Can you work these out from the model? Positions are in its coordinate system, mm. Face numbers are marked on the shaded views. A direction names the side the tool comes from. Give positions to 0.01 mm unless a question says otherwise; leave off trailing zeros. Loops run counter-clockwise (first coordinate to the right, second up) from the corner with the lowest first, then second, coordinate; pieces in that order, holes last. Notation, with made-up numbers: (-33.75, 60.25) - (-17.75, 60.25) arc R16 ccw to (-17.75, 84.25) - close; hole circle Ø3 at (-25.5, 88.25). An arc over 180 degrees is marked (long way). Answer as a JSON object with one key per item and string values. Group by question number.
Item 1: Will these pins go through, and if not, where does the flat tip stop? pin 1 (3 mm diameter, centred on y = 7.5, z = -3.5, fed in from -X); pin 2 (5 mm diameter, centred on x = 14.351, z = 0, fed in from -Y); pin 3 (1 mm diameter, centred on x = -2.5, y = 4, fed in from -Z); pin 4 (2 mm diameter, centred on y = 5.5, z = 5, fed in from +X).
Item 2: Suppose I cut it at C-C on y = 1.5. Count the separate pieces of the cut face and the enclosed holes in it, and give its area (3 significant figures).
Item 3: Please list where these lines run through material, in increasing order: L1, parallel to X at y = 3.75, z = 0; L2, parallel to X at y = 10, z = 6.5; L3, parallel to X at y = 1.5, z = 1.
Item 4: Which directions (+Z, -Z, +X, -X, +Y, -Y) give clear straight access to the entire face, cutting with the end or side of a thin tool? Please do the marked faces 1, 2 and 3.
Item 5: Suppose I cut it at D-D on z = 4. Write out the boundary of the cut face in (x, y), and give its area (3 significant figures).
Item 6: Suppose I cut it at A-A on z = 0. Write out the boundary of the cut face in (x, y), and give its area (3 significant figures).
Item 7: Suppose I cut it at B-B on x = -14. Write out the boundary of the cut face in (y, z), and give its area (3 significant figures).
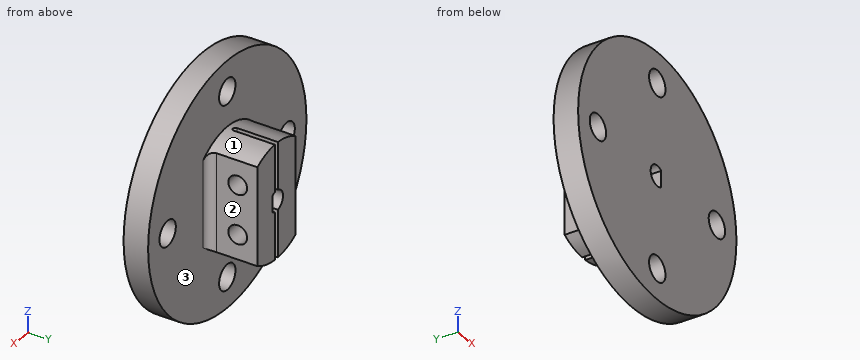
from build123d import *

# Parameters (mm, degrees)
SKETCH1_R               = 19.05
BOSS_EXTRUDE1_DEPTH     = 3.81
SKETCH2_R               = 8.89
BOSS_EXTRUDE2_DEPTH     = 7.62
CUT_EXTRUDE1_DEPTH      = 12.43
CUT_EXTRUDE2_DEPTH      = 20.05
CUT_EXTRUDE2_DEPTH_BACK = 20.05
CUT_EXTRUDE3_DEPTH      = 7.62
FILLET1_R               = 1.27
SKETCH6_R               = 1.4605
CUT_EXTRUDE4_DEPTH      = 24.62905012
SKETCH7_R               = 1.9685
CUT_EXTRUDE5_DEPTH      = 4.8100001


with BuildPart() as part:
    # Sketch1 → Boss-Extrude1 (new body)
    with BuildSketch(Plane(origin=(0, 0, 0), x_dir=(1, 0, 0), z_dir=(0, 1, 0))):
        Circle(SKETCH1_R)
    extrude(amount=BOSS_EXTRUDE1_DEPTH)

    # Sketch2 → Boss-Extrude2 (add)
    with BuildSketch(Plane(origin=(0, 3.81, 0), x_dir=(1, 0, 0), z_dir=(0, 1, 0))):
        Circle(SKETCH2_R)
    extrude(amount=BOSS_EXTRUDE2_DEPTH)

    # Sketch3 → Cut-Extrude1 (cut, through all)
    with BuildSketch(Plane(origin=(0, 11.43, 0), x_dir=(1, 0, 0), z_dir=(0, 1, 0))):
        with BuildLine():
            Line((0.9525, -1.27), (0.9525, 1.27))
            ThreePointArc((0.9525, 1.27), (-1.5875, 0), (0.9525, -1.27))
        make_face()
    extrude(amount=-CUT_EXTRUDE1_DEPTH, mode=Mode.SUBTRACT)

    # Sketch4 → Cut-Extrude2 (cut, two sides)
    with BuildSketch(Plane.XY) as cut_extrude2_sk:
        with BuildLine():
            Line((-0.381, 11.43), (-0.381, 5.08))
            ThreePointArc((-0.381, 5.08), (0, 4.699), (0.381, 5.08))
            Line((0.381, 5.08), (0.381, 11.43))
            Line((0.381, 11.43), (-0.381, 11.43))
        make_face()
    extrude(amount=CUT_EXTRUDE2_DEPTH, mode=Mode.SUBTRACT)
    extrude(cut_extrude2_sk.sketch, amount=-CUT_EXTRUDE2_DEPTH_BACK, mode=Mode.SUBTRACT)

    # Sketch5 → Cut-Extrude3 (cut)
    with BuildSketch(Plane(origin=(0, 11.43, 0), x_dir=(1, 0, 0), z_dir=(0, 1, 0))):
        with BuildLine():
            Line((4.57905012, 7.62), (4.57905012, -7.62))
            ThreePointArc((4.57905012, -7.62), (8.89, 0), (4.57905012, 7.62))
        make_face()
        with BuildLine():
            Line((-4.57905012, -7.62), (-4.57905012, 7.62))
            ThreePointArc((-4.57905012, 7.62), (-8.89, 0), (-4.57905012, -7.62))
        make_face()
    extrude(amount=-CUT_EXTRUDE3_DEPTH, mode=Mode.SUBTRACT)

    # Fillet1
    fillet1_edges = [part.edges().sort_by_distance(p)[0] for p in [
        (4.57905012, 3.81, 0),
        (-4.57905012, 3.81, 0),
    ]]
    fillet(fillet1_edges, radius=FILLET1_R)

    # Sketch6 → Cut-Extrude4 (cut, through all)
    with BuildSketch(Plane(origin=(4.57905012, 0, 0), x_dir=(0, 0, -1), z_dir=(1, 0, 0))):
        with Locations((-3.81, 8.382)):
            Circle(SKETCH6_R)
        with Locations((3.81, 8.382)):
            Circle(SKETCH6_R)
    extrude(amount=-CUT_EXTRUDE4_DEPTH, mode=Mode.SUBTRACT)

    # Sketch7 → Cut-Extrude5 (cut, through all)
    with BuildSketch(Plane(origin=(0, 3.81, 0), x_dir=(1, 0, 0), z_dir=(0, 1, 0))):
        with Locations((-14.2875, 0)):
            Circle(SKETCH7_R)
        with Locations((0, 14.2875)):
            Circle(SKETCH7_R)
        with Locations((14.351, 0)):
            Circle(SKETCH7_R)
        with Locations((0, -14.2875)):
            Circle(SKETCH7_R)
    extrude(amount=-CUT_EXTRUDE5_DEPTH, mode=Mode.SUBTRACT)


solid = part.part
Worked out:
{
 "1": {"pin 1": "stops at x = -4.58", "pin 2": "stops at y = 0", "pin 3": "stops at z = -18.94", "pin 4": "stops at x = 4.72"},
 "2": {"separate pieces": "1", "enclosed holes": "5", "area": "1,080 mm2"},
 "3": {"L1": "x = -19.05 to -16.26, -12.32 to -1.59, 0.95 to 12.38, 16.32 to 19.05", "L2": "x = -4.58 to -0.38, 0.38 to 4.58", "L3": "x = -19.02 to -15.98, -12.59 to -1.23, 0.95 to 12.66, 16.05 to 19.02"},
 "4": {"face 1": "+Z, +Y", "face 2": "+Z, -Z, +X, +Y", "face 3": "+Y"},
 "5": {"outline": "(-18.63, 0) - (18.63, 0) - (18.63, 3.81) - (5.85, 3.81) arc R1.27 cw to (4.58, 5.08) - (4.58, 6.93) - (0.38, 6.93) - (0.38, 5.08) arc R0.38 cw to (-0.38, 5.08) - (-0.38, 6.93) - (-4.58, 6.93) - (-4.58, 5.08) arc R1.27 cw to (-5.85, 3.81) - (-18.63, 3.81) - close; (-4.58, 9.83) - (-0.38, 9.83) - (-0.38, 11.43) - (-4.58, 11.43) - close; (0.38, 9.83) - (4.58, 9.83) - (4.58, 11.43) - (0.38, 11.43) - close", "area": "183 mm2"},
 "6": {"outline": "(-19.05, 0) - (-16.26, 0) - (-16.26, 3.81) - (-19.05, 3.81) - close; (-12.32, 0) - (-1.59, 0) - (-1.59, 11.43) - (-4.58, 11.43) - (-4.58, 5.08) arc R1.27 cw to (-5.85, 3.81) - (-12.32, 3.81) - close; (0.95, 0) - (12.38, 0) - (12.38, 3.81) - (5.85, 3.81) arc R1.27 cw to (4.58, 5.08) - (4.58, 11.43) - (0.95, 11.43) - close; (16.32, 0) - (19.05, 0) - (19.05, 3.81) - (16.32, 3.81) - close", "area": "157 mm2"},
 "7": {"outline": "(0, -12.92) - (3.81, -12.92) - (3.81, -1.95) - (0, -1.95) - close; (0, 1.95) - (3.81, 1.95) - (3.81, 12.92) - (0, 12.92) - close", "area": "83.6 mm2"}
}
